Print and shaded views of the part. All mm, measured from the part's lowest x, y and z. Round coordinates to 2 decimals unless told otherwise and drop trailing zeros. Order: outer loops, then holes, each group sorted by start corner. A loop starts at its lowest first (then second) coordinate and runs counter-clockwise, first axis right, second up. Notation, with made-up numbers: M -36.5,67.25 L -29.5,67.25 A17 cw -29.5,77.25 Z; hole C 10,10.5 d11. An arc over 180 degrees is marked long. Write each question's results on one line, items separated by ' | '. Start each with the question number.
1. Drop flat-ended pins along their axis: pin 1 Ø1 at (y, z) = (21.5, 1) entering from -X; pin 2 Ø1 at (x, z) = (4, 1) entering from +Y (1 decimal). Give the stop position or say it passes through.
2. Band-saw the part on C-C, the plane x = 25.5. List the corners of the cut face in (y, z), then the cut area to 3 significant figures.
3. Probe L1, parallel to Y at x = 14.5, z = 1.5; L2, parallel to X at y = 26.5, z = 0.25 (1 decimal); L3, parallel to X at y = 22.5, z = 1.3. List the from-to ranges inside material, lowest first. Write a range as [from, to].
4. Band-saw the part on A-A, the plane z = 0.3. List the corners of the cut face in (x, y), then the cut area to 3 significant figures.
5. Band-saw the part on B-B, the plane x = 17.5. List the corners of the cut face in (y, z).
6. Band-saw the part on D-D, the plane y = 3. List the corners of the cut face in (x, z).
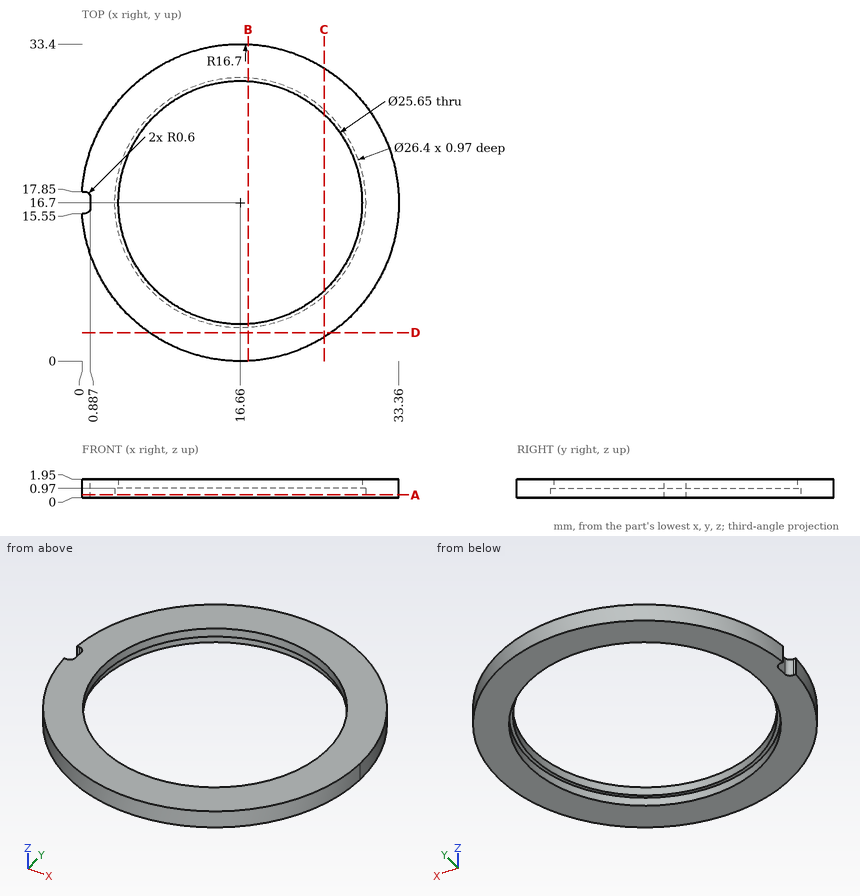
Solution:
1) pin 1: x = 0.52 | pin 2: y = 28.1
2) outline: M 2.53,0 L 6.9,0 L 6.9,0.97 L 7.41,0.97 L 7.41,1.95 L 2.53,1.95 Z; M 25.99,0.97 L 26.5,0.97 L 26.5,0 L 30.87,0 L 30.87,1.95 L 25.99,1.95 Z | area: 18.0 mm^2
3) L1: [0.14, 4.06], [29.34, 33.26] | L2: [3.1, 7.8], [25.5, 30.2] | L3: [1, 5.22], [28.1, 32.32]
4) outline: M 0,15.55 A16.7 ccw long 0,17.85 L 0.29,17.85 A0.6 cw 0.89,17.25 L 0.89,16.15 A0.6 cw 0.29,15.55 Z; hole C 16.66,16.7 d26.4 | area: 327 mm^2
5) outline: M 0.02,0 L 3.53,0 L 3.53,0.97 L 3.9,0.97 L 3.9,1.95 L 0.02,1.95 Z; M 29.5,0.97 L 29.87,0.97 L 29.87,0 L 33.38,0 L 33.38,1.95 L 29.5,1.95 Z
6) outline: M 7.11,0 L 26.21,0 L 26.21,1.95 L 7.11,1.95 Z
